The model under review builds one solid part; all positions refer to its coordinate system, in mm. Face numbers are marked on the shaded views. A direction names the side the tool comes from. Coordinates: 2 decimals unless noted, no trailing zeros. Order: outer loops, then holes, each group sorted by start corner. A loop starts at its lowest first (then second) coordinate and runs counter-clockwise, first axis right, second up. Notation, with made-up numbers: (-38, -30.5) -> (6, -30.5) arc R23 ccw to (6, -18.5) -> close; hole circle Ø10 at (20.25, -25). An arc over 180 degrees is marked (long way). Put each result on its own line as item: value.
from build123d import *

# Parameters (mm, degrees)
SKETCH1_R      = 4
BASE_DEPTH     = 10
POT_HOLE_DEPTH = 8
FILLET1_R      = 0.5


with BuildPart() as part:
    # Sketch1 → Base (new body)
    with BuildSketch(Plane.XY):
        Circle(SKETCH1_R)
    extrude(amount=BASE_DEPTH)

    # Sketch2 → Pot Hole (cut)
    with BuildSketch(Plane(origin=(0, 0, 0), x_dir=(-1, 0, 0), z_dir=(0, 0, -1))):
        with BuildLine():
            Line((-2.598076211, -1.5), (2.598076211, -1.5))
            ThreePointArc((2.598076211, -1.5), (0, 3), (-2.598076211, -1.5))
        make_face()
    extrude(amount=-POT_HOLE_DEPTH, mode=Mode.SUBTRACT)

    # Fillet1
    fillet1_edges = [part.edges().sort_by_distance(p)[0] for p in [
        (-4, 0, 10),
    ]]
    fillet(fillet1_edges, radius=FILLET1_R)


solid = part.part
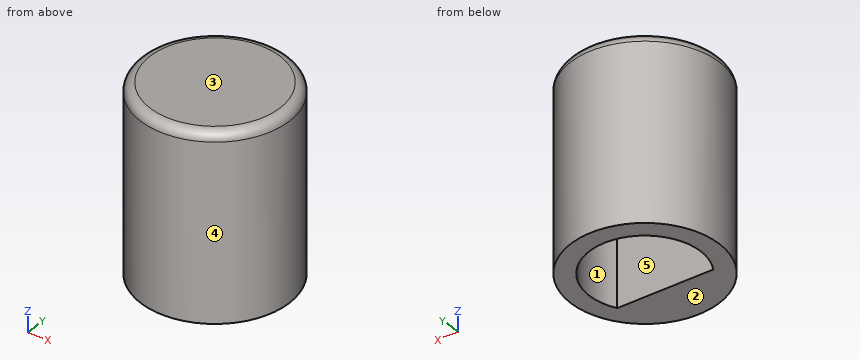
Item 1: For line 1 (Z direction, x = -0.25, y = 1); line 2 (Y direction, x = 1, z = 4); line 3 (Y direction, x = -2.75, z = 2), list the stretches that pass through material, from the lowest coordinate up. Write a range as from..to.
Answers below:
line 1: 8..10
line 2: -3.87..-1.5, 2.83..3.87
line 3: -2.9..-1.2, 1.2..2.9
Item 2: Consider section B-B on x = 0. Write out the cut boundary in (y, z).
Answers below:
outline: (-4, 0) -> (-1.5, 0) -> (-1.5, 8) -> (3, 8) -> (3, 0) -> (4, 0) -> (4, 9.5) arc R0.5 ccw to (3.5, 10) -> (-3.5, 10) arc R0.5 ccw to (-4, 9.5) -> close
Item 3: For pin 1 Ø4 at (x, z) = (3, 2) entering from +Y; pin 2 Ø3 at (y, z) = (1, 6) entering from +X; pin 3 Ø1.5 at (x, z) = (1, 8) entering from -Y; pin 4 Ø2 at (x, y) = (-1, 0) entering from -Z, all flat-tipped, find the tip position at first contact; note any pin that passes through.
Answers below:
pin 1: y = 3.87
pin 2: x = 4
pin 3: y = -3.99
pin 4: z = 8
Item 4: For the marked faces 1 and 2, list the 3-axis set-ups (+Z, -Z, +X, -X, +Y, -Y) from which the entire face can be reached by the end or side of a thin tool; tool diameter is ignored.
Answers below:
face 1: -Z
face 2: -Z, +X, -X, +Y, -Y
Item 5: Consider section C-C on z = 5.75. Write out the cut boundary in (x, y), and give its area (3 significant figures).
Answers below:
outline: circle Ø8 at (0, 0); hole (-2.6, -1.5) -> (2.6, -1.5) arc R3 ccw (long way) to start
area: 27.5 mm^2
Item 6: Consider section A-A on y = 0. Write out the cut boundary in (x, z).
Answers below:
outline: (-4, 0) -> (-3, 0) -> (-3, 8) -> (3, 8) -> (3, 0) -> (4, 0) -> (4, 9.5) arc R0.5 ccw to (3.5, 10) -> (-3.5, 10) arc R0.5 ccw to (-4, 9.5) -> close
Item 7: Mouldability with a two-part tool opening along X and no side actions: class the marked faces 3, 4 and 5 as +X half, -X half, draft (parallel to the pull), parting line (faces both ways), or undercut.
Answers below:
face 3: draft
face 4: parting line
face 5: undercut
